Geometry check sheet. Reference: drawing and pictorial views, mm from the part's lowest x, y, z. Give positions to 0.01 mm unless a question says otherwise; leave off trailing zeros. Write each loop counter-clockwise with the first axis right and the second up, starting at its lowest first coordinate (ties: lowest second). Pieces come first, ordered by that corner, then holes. Notation, with made-up numbers: M 19,22 L 73,22 A16 ccw 73,31 Z; hole C -6.5,33 d4. An arc over 180 degrees is marked long. Answer as a JSON object with one key per item and string values.
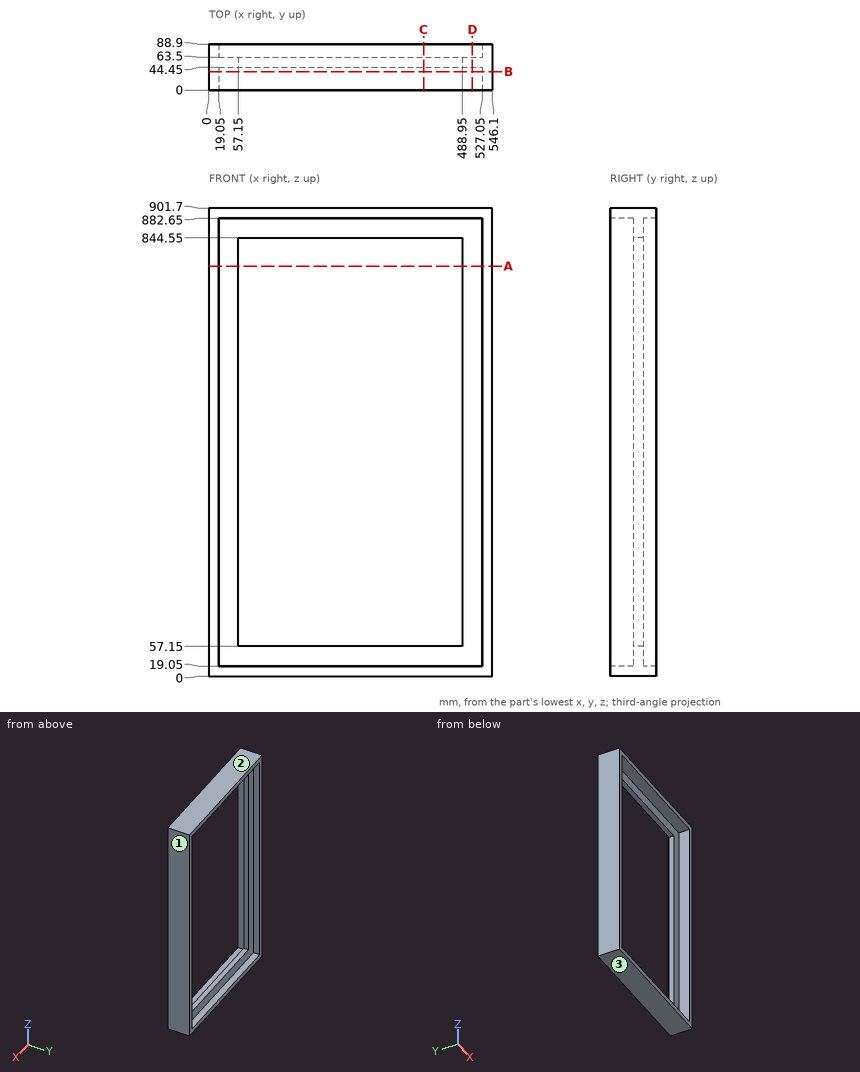
1) Section check C-C on x = 414. Record the boundary of the cut face in (y, z).
Completed:
{"outline": "M 0,0 L 88.9,0 L 88.9,19.05 L 63.5,19.05 L 63.5,57.15 L 44.45,57.15 L 44.45,19.05 L 0,19.05 Z; M 0,882.65 L 44.45,882.65 L 44.45,844.55 L 63.5,844.55 L 63.5,882.65 L 88.9,882.65 L 88.9,901.7 L 0,901.7 Z"}
2) Section check A-A on z = 790. Record the boundary of the cut face in (x, y).
Completed:
{"outline": "M 0,0 L 19.05,0 L 19.05,44.45 L 57.15,44.45 L 57.15,63.5 L 19.05,63.5 L 19.05,88.9 L 0,88.9 Z; M 488.95,44.45 L 527.05,44.45 L 527.05,0 L 546.1,0 L 546.1,88.9 L 527.05,88.9 L 527.05,63.5 L 488.95,63.5 Z"}
3) Thickness scan on L1, parallel to Z at x = 207, y = 82; L2, parallel to Z at x = 235.5, y = 51; L3, parallel to X at y = 21.5, z = 400.5. Record the ranges inside material, lowest first.
Completed:
{"L1": "z = 0 to 19.05, 882.65 to 901.7", "L2": "z = 0 to 57.15, 844.55 to 901.7", "L3": "x = 0 to 19.05, 527.05 to 546.1"}
4) Release check for a two-part mould opening along Z. For the marked faces 1, 2 and 3 record: pulls with the +Z half, pulls with the -Z half, needs draft (parallel to the pull), parting line crosses it, or undercut.
Completed:
{"face 1": "needs draft", "face 2": "pulls with the +Z half", "face 3": "pulls with the -Z half"}
5) Section check D-D on x = 508. Record the boundary of the cut face in (y, z).
Completed:
{"outline": "M 0,0 L 88.9,0 L 88.9,19.05 L 63.5,19.05 L 63.5,882.65 L 88.9,882.65 L 88.9,901.7 L 0,901.7 L 0,882.65 L 44.45,882.65 L 44.45,19.05 L 0,19.05 Z"}
6) Section check B-B on y = 35.5. Record the boundary of the cut face in (x, z), and give its area (3 significant figures).
Completed:
{"outline": "M 0,0 L 546.1,0 L 546.1,901.7 L 0,901.7 Z; hole M 19.05,19.05 L 527.05,19.05 L 527.05,882.65 L 19.05,882.65 Z", "area": "53,700 mm2"}
